Geometry check sheet. Reference: the model listing, model coordinates, mm. A direction names the side the tool comes from. Give positions to 0.01 mm unless a question says otherwise; leave off trailing zeros. Write each loop counter-clockwise with the first axis right and the second up, starting at its lowest first coordinate (ties: lowest second). Pieces come first, ordered by that corner, then holes. Notation, with made-up numbers: (-10.75, -40) - (13.25, -40) arc R8 cw to (13.25, -32) - close; hole circle Ø4 at (10, 61). An arc over 180 degrees is marked (long way). One line per question, with ' | ' between items. Start each with the question number.
Q1. Gauge pin test, flat ends, axial feed: P1, Ø1.5, axis at y = 3, z = 7, coming from the -X side; P2, Ø1.5, axis at y = 0.5, z = 5.5, coming from the +X side; P3, Ø1.5, axis at x = 5, z = 10, coming from the -Y side; P4, Ø1.7, axis at x = 12, z = 1, coming from the +Y side. Record the tip position at first contact, or that the pin passes through.
Q2. Section check B-B on x = 7.5. Record the boundary of the cut face in (y, z), and give its area (3 significant figures).
Q3. Section check D-D on y = 4.6. Record the boundary of the cut face in (x, z), and give its area (3 significant figures).
Q4. Thickness scan on L1, parallel to Y at x = 9, z = 4.5; L2, parallel to Y at x = 13.75, z = 0.75; L3, parallel to X at y = 1.25, z = 12. Record the ranges inside material, lowest first. Write a range as [from, to].
Q5. Set-up check for faces 1 (the face through (2, 3, 13)), 2 (the face through (8.371, 4.24, 5.153)), 3 (the face through (12.285, 3.246, 1.558)), 4 (the face through (0.74, 1.48, 13.36)): record each of +Z, -Z, +X, -X, +Y, -Y from which the full face is reachable in a straight line by a thin tool's end or side.
Q6. Section check A-A on z = 7.25. Record the boundary of the cut face in (x, y).
Q7. Section check C-C on y = 1.55. Record the boundary of the cut face in (x, z).
```python
from build123d import *

# Parameters (mm, degrees)
SKETCH1_R             = 2
BOSS_EXTRUDE1_DEPTH   = 3
BOSS_EXTRUDE1_2_DEPTH = 3
BOSS_EXTRUDE2_DEPTH   = 4
SKETCH4_R             = 2
BOSS_EXTRUDE3_DEPTH   = 1.5


with BuildPart() as part:
    # Sketch1 → Boss-Extrude1 (new body)
    with BuildSketch(Plane(origin=(0, 0, 0), x_dir=(1, 0, 0), z_dir=(0, 1, 0))):
        with Locations((2.326314278, -12.139796801)):
            Circle(SKETCH1_R)
    extrude(amount=BOSS_EXTRUDE1_DEPTH)



with BuildPart() as body_2:
    # Sketch1 → Boss-Extrude1 2 (new body)
    with BuildSketch(Plane(origin=(0, 0, 0), x_dir=(1, 0, 0), z_dir=(0, 1, 0))):
        with Locations((12.264503501, -1.538947167)):
            Circle(SKETCH1_R)
    extrude(amount=BOSS_EXTRUDE1_2_DEPTH)


with BuildPart() as part_1:
    add(part.part)

    add(body_2.part)  # Boss-Extrude2 merges body 2
    # Sketch2 → Boss-Extrude2 (add)
    with BuildSketch(Plane(origin=(8.754490667, 0, 8.207246381), x_dir=(0.683937198, 0, -0.729540889), z_dir=(0.729540889, 0, 0.683937198))):
        Polygon((5.26542528, 3), (7.26542528, 3), (7.26542528, 3.5), (-7.26542528, 3.5), (-7.26542528, 3), align=None)
        Polygon((7.26542528, 2.5), (7.26542528, 3), (5.26542528, 3), (-7.26542528, 3), (-7.26542528, 2.5), align=None)
    extrude(amount=-BOSS_EXTRUDE2_DEPTH)

    # Sketch4 → Boss-Extrude3 (add)
    with BuildSketch(Plane(origin=(0, 3.5, 0), x_dir=(1, 0, 0), z_dir=(0, 1, 0))):
        with Locations((7.295408889, -6.839371984)):
            Circle(SKETCH4_R)
    extrude(amount=BOSS_EXTRUDE3_DEPTH)


solid = part_1.part
```
Working result:
1) P1: stops at x = 3.7 | P2: passes through | P3: stops at y = 2.5 | P4: stops at y = 3.5
2) outline: (2.5, 3.7) - (3.5, 3.7) - (3.5, 4.85) - (5, 4.85) - (5, 8.83) - (3.5, 8.83) - (3.5, 9.55) - (2.5, 9.55) - close | area: 11.8 mm2
3) outline: circle Ø4 at (7.3, 6.84) | area: 12.6 mm2
4) L1: y = [2.5, 3.5] | L2: y = [0, 3] | L3: x = [0.33, 4.32]
5) face 1: +Z, -X, +Y | face 2: +Y | face 3: -Z, +X, +Y | face 4: -Y
6) outline: (4.17, 2.5) - (9.65, 2.5) - (9.65, 3.5) - (9.25, 3.5) - (9.25, 5) - (5.34, 5) - (5.34, 3.5) - (4.17, 3.5) - close
7) outline: circle Ø4 at (2.33, 12.14); circle Ø4 at (12.26, 1.54)
